```python
from build123d import *

# Parameters (mm, degrees)
F0_R     = 4.7625
F1_DEPTH = 5.95122
F2_DEPTH = 38.1
F3_SIZE  = 0.508
F4_SIZE  = 0.508


with BuildPart() as f1:
    # F0 (on Top) → F1 (new body)
    with BuildSketch(Plane.XY):
        Polygon((7.14375, -4.124446), (7.14375, 4.124446), (0, 8.248892), (-7.14375, 4.124446), (-7.14375, -4.124446), (0, -8.248892), align=None)
        Circle(F0_R, mode=Mode.SUBTRACT)
        Circle(F0_R)
    extrude(amount=F1_DEPTH)

    # F0 (on Top) → F2 (join)
    with BuildSketch(Plane.XY):
        Circle(F0_R)
    extrude(amount=-F2_DEPTH)

    # F3
    f3_edges = [f1.edges().sort_by_distance(p)[0] for p in [
        (-4.7625, 0, -38.1),
    ]]
    chamfer(f3_edges, length=F3_SIZE)

    # F4
    f4_edges = [f1.edges().sort_by_distance(p)[0] for p in [
        (3.571875, -6.186669, 5.95122),
        (7.14375, 0, 5.95122),
        (3.571875, 6.186669, 5.95122),
        (-3.571875, 6.186669, 5.95122),
        (-7.14375, 0, 5.95122),
        (-3.571875, -6.186669, 5.95122),
        (-3.571875, -6.186669, 0),
        (3.571875, -6.186669, 0),
        (7.14375, 0, 0),
        (-7.14375, 0, 0),
        (-3.571875, 6.186669, 0),
    ]]
    chamfer(f4_edges, length=F4_SIZE)


solid = f1.part
```
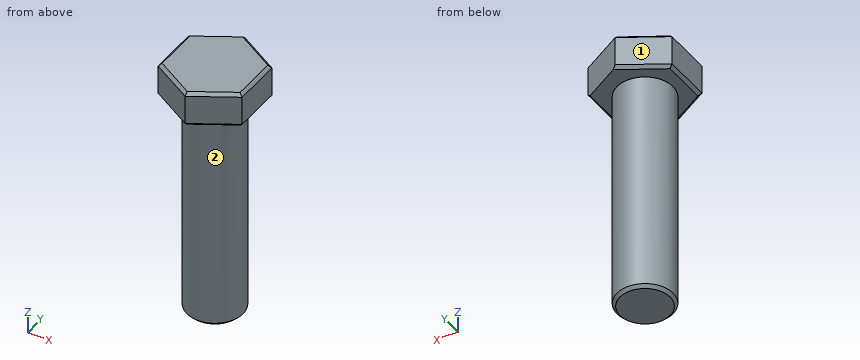
Read the model definition and answer for the solid it produces. Units are mm, in the model's axes. Face numbers are marked on the shaded views. A direction names the side the tool comes from. Give positions to 0.01 mm unless a question says otherwise; leave off trailing zeros. Write each loop counter-clockwise with the first axis right and the second up, starting at its lowest first coordinate (ties: lowest second). Pieces come first, ordered by that corner, then holes. Notation, with made-up numbers: (-1.75, -25) - (17.25, -25) arc R23 ccw to (17.25, 8) - close; hole circle Ø11 at (60.5, -35). An arc over 180 degrees is marked (long way). Write item = value, one per line. Start each with the question number.
Item 1: A tool of negligible diameter and unlimited length cuts with its end or side. For the marked faces 1 and 2, from which of +Z, -Z, +X, -X, +Y, -Y can it reach the whole face along a straight path? Write none if from no direction.
Item 2: Find section A-A (y = 0). Give the vertices of the cut face in (x, z).
Item 3: Find section B-B (z = -8). Give the vertices of the cut face in (x, y) (1 decimal).
Item 4: Find the intervals of material crossed by probe 1 along Z at (x, y) = (6, 0.25); probe 2 along Y at (x, z) = (4, -0.5); probe 3 along Y at (x, z) = (-4.25, -12), in increasing order. Write a range as [from, to].
Item 5: Find section C-C (x = -5.25). Give the vertices of the cut face in (y, z), then the cut area to 3 significant figures.
Item 6: Find section D-D (y = 6.75). Give the vertices of the cut face in (x, z), then the cut area to 3 significant figures.
Item 7: Each of these flat-tipped pins is pushed along its axis until it touches: P1, Ø2, axis at y = 4.5, z = -7.5, coming from the -X side; P2, Ø2, axis at x = -4.5, z = -21.5, coming from the -Y side; P3, Ø4, axis at x = -2, y = -6.5, coming from the -Z side. Where does it stop, or does it pass through?
Response:
q1.face_1 = +Z, -Z, -X, +Y
q1.face_2 = -Z
q2.outline = (-7.14, 0.51) - (-6.64, 0) - (-4.76, 0) - (-4.76, -37.59) - (-4.25, -38.1) - (4.25, -38.1) - (4.76, -37.59) - (4.76, 0) - (6.64, 0) - (7.14, 0.51) - (7.14, 5.44) - (6.64, 5.95) - (-6.64, 5.95) - (-7.14, 5.44) - close
q3.outline = circle Ø9.5 at (0, 0)
q4.probe_1 = [0, 5.95]
q4.probe_2 = [-2.58, 2.58]
q4.probe_3 = [-2.15, 2.15]
q5.outline = (-5.22, 0.51) - (-4.63, 0) - (4.63, 0) - (5.22, 0.51) - (5.22, 5.44) - (4.63, 5.95) - (-4.63, 5.95) - (-5.22, 5.44) - close
q5.area = 61.5 mm²
q6.outline = (-2.6, 0.51) - (-1.58, 0) - (2.6, 0) - (2.6, 5.44) - (1.58, 5.95) - (-1.58, 5.95) - (-2.6, 5.44) - close
q6.area = 30.1 mm²
q7.P1 = -3.23
q7.P2 = -3.23
q7.P3 = 0
